Part model, mm, in its own coordinate system. Face numbers are marked on the shaded views. A direction names the side the tool comes from. Round coordinates to 2 decimals unless told otherwise and drop trailing zeros. Write each loop counter-clockwise with the first axis right and the second up, starting at its lowest first coordinate (ties: lowest second). Pieces come first, ordered by that corner, then holes. Notation, with made-up numbers: (62, -40) -> (107, -40) arc R18 cw to (107, -29) -> close; hole circle Ø7 at (51, -9). An arc over 180 degrees is marked (long way). Return JSON: item names as keys, results as strings. Group by question number.
(1) Mould opens along X. For the marked faces 3, 4 and 5 say: +X half, -X half, draft (parallel to the pull), parting line (faces both ways), or undercut.
(2) Saw through at C-C (x = 5). List the corners of the cut face in (y, z).
(3) Saw through at A-A (y = 0). List the corners of the cut face in (x, z).
(4) Tool access for the marked faces 1 and 2: list every direction of +Z, -Z, +X, -X, +Y, -Y with a clear straight run to the whole face (end or side of a thin tool).
(5) Drill centre lines: L1, parallel to X at y = 0, z = 1.1; L2, parallel to X at y = 1.5, z = -2; L3, parallel to Y at x = 71.5, z = 1. Where is each one in solid material? Low to high. Write a range as from..to.
(6) Drop flat-ended pins along their axis: pin 1 Ø1 at (x, z) = (16.5, -0.5) entering from -Y; pin 2 Ø3 at (y, z) = (-16, 1) entering from +X; pin 3 Ø1.5 at (y, z) = (-7, -2.5) entering from +X. Give the stop position or say it passes through.
(7) Saw through at B-B (z = -1.5). List the corners of the cut face in (x, y), plus the area to 3 significant figures.
Autodesk Inventor part; units mm, degrees
ref_plane "YZ Plane" through (0, 0, 0) normal (1, 0, 0) x (0, 1, 0)
ref_plane "XZ Plane" through (0, 0, 0) normal (0, 1, 0) x (-1, 0, 0)
ref_plane "XY Plane" through (0, 0, 0) normal (0, 0, 1) x (1, 0, 0)
sketch "Sketch1" plane through (0, 0, 0) normal (0, 0, 1) x (1, 0, 0)
  arc A0 (-1.4131, 5.8312) -> (-1.4131, -5.8312) centre (0, 0) ccw
  arc A1 (58.7458, -20.4093) -> (58.7458, 20.4093) centre (63.6915, 0) ccw
  line L0 (-1.4131, 5.8312) -> (58.7458, 20.4093)
  line L1 (-1.4131, -5.8312) -> (58.7458, -20.4093)
  line L2 (58.4396, 21.6727) -> (-1.7192, 7.0947)
  arc A2 (-1.7192, 7.0947) -> (-1.7192, -7.0947) centre (0, 0) ccw
  line L3 (-1.7192, -7.0947) -> (58.4396, -21.6727)
  arc A3 (58.4396, -21.6727) -> (58.4396, 21.6727) centre (63.6915, 0) ccw
  dimension "d0" = 12
  dimension "d1" = 42
  dimension "d2" = 61.9
  dimension "d3" = 1.3
extrude "Extrusion1" add sketch "Sketch1" along normal mid plane 6
chamfer "Chamfer1" distance 0.5 angle 45 8 edges at (-6, 0, 3) (28.6664, 13.1203, 3) (84.6915, 0, 3) (28.6664, -13.1203, 3) (-6, 0, -3) (28.6664, -13.1203, -3) (84.6915, 0, -3) (28.6664, 13.1203, -3)
properties part number "Tandriem20naar60T" material "Rubber"
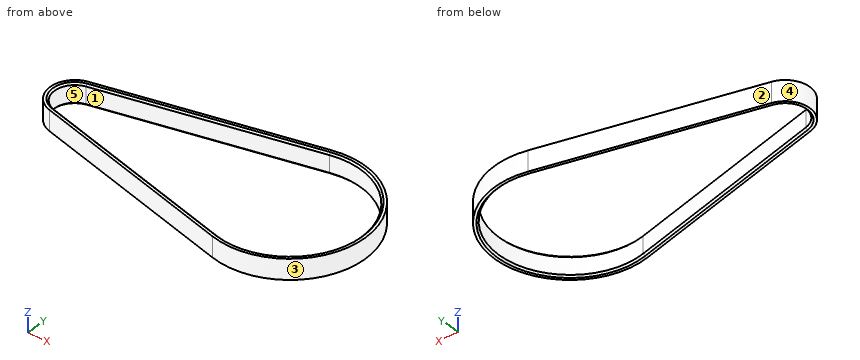
Computed values:
{
 "1": {"face 3": "parting line", "face 4": "-X half", "face 5": "undercut"},
 "2": {"outline": "(-8.72, -3) -> (-7.9, -3) -> (-7.39, -2.5) -> (-7.39, 2.5) -> (-7.9, 3) -> (-8.72, 3) -> close; (7.39, -2.5) -> (7.9, -3) -> (8.72, -3) -> (8.72, 3) -> (7.9, 3) -> (7.39, 2.5) -> close"},
 "3": {"outline": "(-7.3, -3) -> (-6.5, -3) -> (-6, -2.5) -> (-6, 2.5) -> (-6.5, 3) -> (-7.3, 3) -> close; (84.69, -2.5) -> (85.19, -3) -> (85.99, -3) -> (85.99, 3) -> (85.19, 3) -> (84.69, 2.5) -> close"},
 "4": {"face 1": "+Z, -Z", "face 2": "+Z, -Z, -X, +Y"},
 "5": {"L1": "-7.3..-6, 84.69..85.99", "L2": "-7.14..-5.81, 84.64..85.94", "L3": "-20.89..-19.49, 19.49..20.89"},
 "6": {"pin 1": "y = -11.63", "pin 2": "x = 80.63", "pin 3": "x = 85.1"},
 "7": {"outline": "(-1.72, -7.09) -> (58.44, -21.67) arc R22.3 ccw (long way) to (58.44, 21.67) -> (-1.72, 7.09) arc R7.3 ccw to start; hole (-1.41, -5.83) -> (58.75, -20.41) arc R21 ccw (long way) to (58.75, 20.41) -> (-1.41, 5.83) arc R6 ccw to start", "area": "286 mm2"}
}
